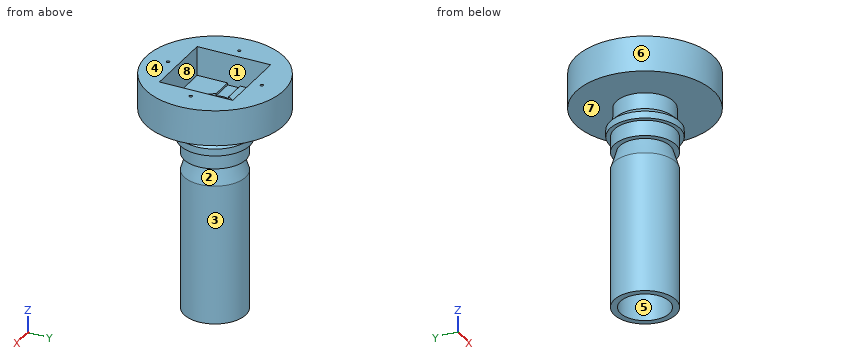
Autodesk Fusion 360 part; units mm, degrees
sketch "Sketch1" plane through (0, 0, 0) normal (0, 0, 1) x (1, 0, 0) in component "Arm Cam"
  circle A0 centre (0, 0) radius 14.75
  circle A1 centre (0, 0) radius 11.75
  dimension "d322" = 29.5
  dimension "d323" = -3
  dimension "d395" = 23.5
extrude "Extrude1" add sketch "Sketch1" along normal blind 67.1 makes body 1 in component "Arm Cam"
sketch "Sketch5" plane through (0, 0, 67.1) normal (0, 0, 1) x (-1, 0, 0) in component "Arm Cam"
  circle A0 centre (0, 0) radius 11.75
  circle A1 centre (0, 0) radius 14.75
  circle A2 centre (0, 0) radius 14.75
ref_plane "WorkPlane2" through (0, 0, 75.5) normal (0, 0, 1) x (1, 0, 0) in component "Arm Cam"
sketch "Sketch4" plane through (-143.4796, -223.0695, 75.5) normal (0, 0, 1) x (1, 0, 0) in component "Arm Cam"
  circle A0 centre (143.4796, 223.0695) radius 14.75
  circle A1 centre (143.4796, 223.0695) radius 12.15
  point P0 (143.4796, 223.0695)
  dimension "d330" = 29.5
  dimension "d334" = 24.3
loft "Loft2" add profiles "Sketch5", "Sketch4" section 1 section 2 contours A1 bodies 1 in component "Arm Cam"
extrude "Extrude4" add sketch "Sketch4" along normal blind 7.4 contours A0 | A1 bodies 1 in component "Arm Cam"
sketch "Sketch7" plane through (0, 0, 82.9) normal (0, 0, 1) x (-1, 0, 0) in component "Arm Cam"
  circle A0 centre (0, 0) radius 14.75
  circle A1 centre (0, 0) radius 16.75
  dimension "d339" = 33.5
extrude "Extrude5" add sketch "Sketch7" along normal blind 3.35 contours A0 | A1 bodies 1 in component "Arm Cam"
ref_plane "WorkPlane3" through (0, 0, 89.15) normal (0, 0, 1) x (-1, 0, 0) in component "Arm Cam"
sketch "Sketch8" plane through (-143.4796, -223.0695, 89.15) normal (0, 0, 1) x (1, 0, 0) in component "Arm Cam"
  circle A0 centre (143.4796, 223.0695) radius 13.75
  point P0 (143.4796, 223.0695)
  dimension "d341" = 27.5
extrude "Extrude6" add sketch "Sketch8" along normal blind 7.7 separate body makes body 2 in component "Arm Cam"
loft "Loft3" add section 1 face at (-0.9963, -4.3652, 86.25) section 2 face at (-1.0199, 5.8346, 89.15) on bodies 1 2 bodies 1 2 in component "Arm Cam"
sketch "Sketch9" plane through (0, 0, 96.85) normal (0, 0, 1) x (-1, 0, 0) in component "Arm Cam"
  circle A0 centre (0, 0) radius 13.75
  circle A1 centre (0, 0) radius 33
  dimension "d344" = 66
  dimension "d351" = 27.5
extrude "Extrude7" add sketch "Sketch9" along normal blind 17 contours A0 | A1 bodies 1 in component "Arm Cam"
sketch "Sketch10" plane through (0, 0, 113.85) normal (0, 0, 1) x (-1, 0, 0) in component "Arm Cam"
  circle A0 centre (0, 0) radius 33
  line L0 (-17.6, 17.6) -> (17.6, 17.6)
  line L1 (17.6, 17.6) -> (17.6, -17.6)
  line L2 (17.6, -17.6) -> (-17.6, -17.6)
  line L3 (-17.6, -17.6) -> (-17.6, 17.6)
  line L4 (-17.6, 17.6) -> (17.6, -17.6) construction
  line L5 (17.6, 17.6) -> (-17.6, -17.6) construction
  circle A1 centre (0, 0) radius 7.5
  line L6 (-17.6, 3) -> (17.6, 3)
  line L7 (17.6, 3) -> (17.6, -3)
  line L8 (17.6, -3) -> (-17.6, -3)
  line L9 (-17.6, -3) -> (-17.6, 3)
  line L10 (-17.6, 3) -> (17.6, -3) construction
  line L11 (17.6, 3) -> (-17.6, -3) construction
  line L12 (-22.5, 22.5) -> (22.5, 22.5) construction
  line L13 (22.5, 22.5) -> (22.5, -22.5) construction
  line L14 (22.5, -22.5) -> (-22.5, -22.5) construction
  line L15 (-22.5, -22.5) -> (-22.5, 22.5) construction
  line L16 (-22.5, 22.5) -> (22.5, -22.5) construction
  line L17 (22.5, 22.5) -> (-22.5, -22.5) construction
  circle A2 centre (22.5, 0) radius 0.75
  circle A3 centre (0, -22.5) radius 0.75
  circle A4 centre (-22.5, 0) radius 0.75
  circle A5 centre (0, 22.5) radius 0.75
  dimension "d347" = 35.2
  dimension "d348" = 35.2
  dimension "d352" = 15
  dimension "d354" = 6
  dimension "d357" = 45
  dimension "d358" = 45
  dimension "d359" = 1.5
  dimension "d360" = 1.5
  dimension "d361" = 1.5
  dimension "d362" = 1.5
extrude "Extrude8" cut sketch "Sketch10" against normal blind 14 contours L0 L1 L3 A1 L6 | L3 A1 L6 L8 L9 | L1 A1 L6 L7 L8 | L1 L2 L3 A1 L8 | A1 L6 L8 | A1 L6 | A1 L8 bodies 1 in component "Arm Cam"
extrude "Extrude9" cut sketch "Sketch10" against normal through all contours A1 L6 L8 | A1 L6 | A1 L8 bodies 1 1 in component "Arm Cam"
extrude "Extrude10" cut sketch "Sketch10" against normal blind 15 contours L3 A1 L6 L8 L9 | L1 A1 L6 L7 L8 bodies 1 in component "Arm Cam"
extrude "Extrude11" cut sketch "Sketch10" against normal blind 10 contours A2 | A3 | A4 | A5 bodies 1 in component "Arm Cam"
component "Arm Cam" placed x (1, 0, 0) y (0, 1, 0) z (0, 0, 1) at (0, 0, 0)
equation "Trous_Vis_diam2 = 2.2 mm"
The model under review builds one solid part; all positions refer to its coordinate system, in mm. Face numbers are marked on the shaded views. A direction names the side the tool comes from. Round coordinates to 2 decimals unless told otherwise and drop trailing zeros. Order: outer loops, then holes, each group sorted by start corner. A loop starts at its lowest first (then second) coordinate and runs counter-clockwise, first axis right, second up. Notation, with made-up numbers: (31.25, 63.5) -> (75.25, 63.5) arc R26 cw to (75.25, 92.5) -> close; hole circle Ø7 at (57.5, 53). An arc over 180 degrees is marked (long way). Write item = value, one per line. Start each with the question number.
Item 1: Mouldability with a two-part tool opening along Y and no side actions: class the marked faces 5, 6, 7 and 8 as released by +Y, released by -Y, zero draft, split by the parting line, or undercut.
Item 2: For the marked faces 1, 2, 3 and 4, list the 3-axis set-ups (+Z, -Z, +X, -X, +Y, -Y) from which the entire face can be reached by the end or side of a thin tool; tool diameter is ignored.
Item 3: Consider section A-A on z = 59.5. Write out the cut boundary in (x, y).
Item 4: For line 1 along Y through (x, z) = (0, 111); line 2 along Y through (x, z) = (0, 22); line 3 along Y through (x, z) = (0, 78), list the stretches that pass through material, from the lowest coordinate up.
Item 5: Consider section B-B on y = 28. Write out the cut boundary in (x, z).
Item 6: Consider section C-C on z = 93. Write out the cut boundary in (x, y).
Item 7: Clearance check with flat-ended pins moving along their axes: pin 1 Ø6 at (x, z) = (3, 97.5) entering from +Y; pin 2 Ø4 at (x, y) = (-13, 14) entering from +Z; pin 3 Ø10 at (y, z) = (-16, 44) entering from +X; pin 4 Ø4 at (x, z) = (-18, 93) entering from -Y. State where each tip first meets the part, or that it passes through.
Conclusion:
q1.face_5 = undercut
q1.face_6 = split by the parting line
q1.face_7 = zero draft
q1.face_8 = undercut
q2.face_1 = +Z
q2.face_2 = none
q2.face_3 = -Z
q2.face_4 = +Z, +X, -X, +Y, -Y
q3.outline = circle Ø29.5 at (0, 0); hole circle Ø23.5 at (0, 0)
q4.line_1 = -33 to -23.25, -21.75 to -17.6, 17.6 to 21.75, 23.25 to 33
q4.line_2 = -14.75 to -11.75, 11.75 to 14.75
q4.line_3 = -14.75 to -7.5, 7.5 to 14.75
q5.outline = (-17.46, 96.85) -> (17.46, 96.85) -> (17.46, 113.85) -> (-17.46, 113.85) -> close
q6.outline = circle Ø27.5 at (0, 0); hole circle Ø15 at (0, 0)
q7.pin_1 = 33
q7.pin_2 = 99.85
q7.pin_3 = 9.83
q7.pin_4 = through
